Geometry check sheet. Reference: the model listing, model coordinates, mm. A direction names the side the tool comes from. Coordinates: 2 decimals unless noted, no trailing zeros. Order: outer loops, then holes, each group sorted by start corner. A loop starts at its lowest first (then second) coordinate and runs counter-clockwise, first axis right, second up. Notation, with made-up numbers: (-27.5, 8.25) - (29.5, 8.25) arc R24 cw to (29.5, 19.25) - close; hole circle Ø10 at (76.25, -25.5). An arc over 180 degrees is marked (long way). Return JSON: item names as keys, results as strings. Group by question number.
Item 1: Tool access check on faces 4 (the flat face through (-18, 5, 5)), 5 (the flat face through (0, 10, 3)), 6 (the flat face through (2, -3, 4.5)). Record the directions out of +Z, -Z, +X, -X, +Y, -Y that give a thin tool (end or side, any length) a straight path to the whole face; none if there is none.
Item 2: Section check B-B on z = 1.05. Enter the section's corners in (x, y), then the cut area to 3 significant figures.
Item 3: Scan lines: probe 1 along X at (y, z) = (5, 1.85); probe 2 along Y at (x, z) = (13.5, 1.4); probe 3 along Z at (x, y) = (16, 0.5). Record each from-to range of solid material in increasing order.
Item 4: Section check C-C on y = 3.75. Give the number of separate pieces and of enclosed holes in the cut face, then the cut area to 3 significant figures.
Item 5: Draft check along X on faces 1 (the flat face through (-18, -3, 4.5)), 2 (the flat face through (13.48, -3.46, 3.51)), 3 (the flat face through (18.48, -2.61, 3.51)). Enter one of: pulls with the +X half, pulls with the -X half, needs draft (parallel to the pull), parting line crosses it, or undercut.
Item 6: Section check A-A on z = 5. Enter the section's corners in (x, y).
Item 7: Gauge pin test, flat ends, axial feed: pin 1 (1.2 mm diameter, centred on x = 15.5, y = -3.5, fed in from +Z); pin 2 (3 mm diameter, centred on x = 4.5, y = -4, fed in from +Z); pin 3 (5.5 mm diameter, centred on x = 13.5, y = 5, fed in from -Z); pin 4 (1 mm diameter, centred on x = 4, z = 5, fed in from -Y). Record the tip position at first contact, or that the pin passes through.
from build123d import *

# Parameters (mm, degrees)
SKETCH_1_W             = 40
SKETCH_1_H             = 20
SKETCH_1_R             = 1.75
EXTRUDE_1_DEPTH        = 6
SKETCH_2_W             = 40
SKETCH_2_H             = 1.5
CUT_EXTRUDE_1_DEPTH    = 15
CUT_EXTRUDE_2_DEPTH    = 15
PATTERN_LINEAR_1_COUNT = 8
PATTERN_LINEAR_1_PITCH = 5


with BuildPart() as part:
    # 草圖1 → 填料-伸長1 (new body)
    with BuildSketch(Plane.XY):
        Rectangle(SKETCH_1_W, SKETCH_1_H)
        with Locations((-13.5, 5)):
            Circle(SKETCH_1_R, mode=Mode.SUBTRACT)
        with Locations((13.5, 5)):
            Circle(SKETCH_1_R, mode=Mode.SUBTRACT)
    extrude(amount=EXTRUDE_1_DEPTH)

    # 草圖2 → 除料-伸長1 (cut)
    with BuildSketch(Plane.XZ.offset(10)):
        with Locations((0, 5.25)):
            Rectangle(SKETCH_2_W, SKETCH_2_H)
    extrude(amount=-CUT_EXTRUDE_1_DEPTH, mode=Mode.SUBTRACT)

    # 草圖3 → 除料-伸長2 (cut)
    with BuildSketch(Plane(origin=(0, -10, 0), x_dir=(-1, 0, 0), z_dir=(0, -1, 0))):
        Polygon((20, -4.5), (18.214101615, -4.5), (18.75, -2.5), (20, -2.5), align=None)
        Polygon((16.785898385, -4.5), (16.25, -2.5), (15, -2.5), (15, -4.5), align=None)
    cut_extrude_2 = extrude(amount=-CUT_EXTRUDE_2_DEPTH, mode=Mode.SUBTRACT)

    # 直線複製排列1: 除料-伸長2 ×8
    with Locations(*[(i * PATTERN_LINEAR_1_PITCH, 0, 0) for i in range(1, PATTERN_LINEAR_1_COUNT)]):
        add(cut_extrude_2, mode=Mode.SUBTRACT)


solid = part.part
Computed:
{
 "1": {"face 4": "+Z, -Y", "face 5": "+Z, -Z, +X, -X, +Y", "face 6": "+Z, +X, -X, -Y"},
 "2": {"outline": "(-20, -10) - (20, -10) - (20, 10) - (-20, 10) - close; hole circle Ø3.5 at (-13.5, 5); hole circle Ø3.5 at (13.5, 5)", "area": "781 mm²"},
 "3": {"probe 1": "x = -20 to -15.25, -11.75 to 11.75, 15.25 to 20", "probe 2": "y = -10 to 3.25, 6.75 to 10", "probe 3": "z = 0 to 2.5"},
 "4": {"separate pieces": "3", "enclosed holes": "0", "area": "114 mm²"},
 "5": {"face 1": "needs draft", "face 2": "undercut", "face 3": "pulls with the +X half"},
 "6": {"outline": "(-20, 5) - (-15.25, 5) arc R1.75 cw to (-11.75, 5) - (11.75, 5) arc R1.75 cw to (15.25, 5) - (20, 5) - (20, 10) - (-20, 10) - close"},
 "7": {"pin 1": "stops at z = 2.5", "pin 2": "stops at z = 4.5", "pin 3": "stops at z = 0", "pin 4": "stops at y = 5"}
}
